Geometry check sheet. Reference: the model listing, model coordinates, mm. Face numbers are marked on the shaded views. A direction names the side the tool comes from. Coordinates: 2 decimals unless noted, no trailing zeros. Loops run counter-clockwise (first coordinate to the right, second up) from the corner with the lowest first, then second, coordinate; pieces in that order, holes last. Notation, with made-up numbers: M 66.25,77.25 L 112.25,77.25 A14 ccw 112.25,88.25 Z; hole C 64.25,87 d10. An arc over 180 degrees is marked long. Use CSV: the item, a comma, the result in double quotes.
Autodesk Fusion 360 part; units mm, degrees
sketch "mainBase" plane through (0, 0, 0) normal (0, 0, 1) x (1, 0, 0)
  line L0 (0, 0) -> (13.7, 0)
  line L1 (13.7, 0) -> (13.7, 6)
  line L2 (13.7, 6) -> (0, 6)
  line L3 (0, 6) -> (0, 0)
  line L4 (0, 0) -> (6.85, 0)
  line L5 (6.85, 0) -> (6.85, 1.75)
  line L6 (6.85, 1.75) -> (1.85, 1.75)
  line L7 (6.85, 1.75) -> (11.85, 1.75)
  line L8 (0, 6) -> (6.85, 6)
  circle A0 centre (1.85, 1.75) radius 1
  circle A1 centre (11.85, 1.75) radius 1
  line L9 (6.85, 6) -> (3.35, 6)
  line L10 (3.35, 6) -> (3.35, 2)
  line L11 (3.35, 2) -> (6.85, 2)
  line L12 (6.85, 2) -> (6.85, 6)
  line L13 (6.85, 6) -> (10.35, 6)
  line L14 (10.35, 6) -> (10.35, 2)
  line L15 (10.35, 2) -> (6.85, 2)
  line L16 (6.85, 2) -> (6.85, 6)
  dimension "d9" = 6
  dimension "d10" = 13.7
  dimension "d11" = 6.85
  dimension "d12" = 1.75
  dimension "d13" = 5
  dimension "d14" = 5
  dimension "d15" = 6.85
  dimension "d17" = 2
  dimension "d18" = 2
  dimension "d19" = 4
  dimension "d20" = 3.5
  dimension "d21" = 4
  dimension "d22" = 3.5
extrude "Extrude1" add sketch "mainBase" along normal blind 7.6 contours L2 L8 L9 L10 L11 L12 L16 | L2 L12 L13 L14 L15 L16
shell "Shell1" thickness 1 removed faces 1 at (5.6833, 4.6667, 0)
extrude "Extrude2" add sketch "mainBase" along normal blind 2 contours L0 L1 L2 L3 L4 L8 L10 L11 L14 L15
sketch "hallCutOut" plane through (0, 0, 0) normal (0, 0, 1) x (1, 0, 0)
  line L0 (0, 6) -> (6.85, 6)
  line L1 (6.85, 6) -> (6.85, 2)
  line L2 (6.85, 2) -> (3.35, 2)
  line L3 (3.35, 2) -> (3.35, 4)
  line L4 (6.85, 2) -> (6.85, 3)
  line L5 (6.85, 3) -> (5.95, 3)
  line L6 (5.95, 3) -> (3.35, 4)
  line L7 (6.85, 3) -> (7.75, 3)
  line L8 (6.85, 2) -> (10.35, 2)
  line L9 (10.35, 2) -> (10.35, 4)
  line L10 (10.35, 4) -> (7.75, 3)
  line L11 (7.75, 3) -> (9.35, 3)
  line L12 (9.35, 3) -> (9.35, 3.6154)
  line L13 (5.95, 3) -> (4.35, 3)
  line L14 (4.35, 3) -> (4.35, 3.6154)
  line L15 (6.85, 5) -> (8.95, 5)
  line L16 (8.95, 5) -> (8.95, 3)
  line L17 (8.95, 3) -> (6.85, 3)
  line L18 (6.85, 3) -> (6.85, 5)
  line L19 (6.85, 5) -> (4.75, 5)
  line L20 (4.75, 5) -> (4.75, 3)
  line L21 (4.75, 3) -> (6.85, 3)
  line L22 (6.85, 3) -> (6.85, 5)
  line L23 (9.35, 3) -> (4.35, 3)
  line L24 (4.35, 3) -> (4.35, 5)
  line L25 (4.35, 5) -> (9.35, 5)
  line L26 (9.35, 5) -> (9.35, 3)
  dimension "d31" = 6.85
  dimension "d32" = 4
  dimension "d33" = 3.5
  dimension "d34" = 2
  dimension "d35" = 1
  dimension "d36" = 0.9
  dimension "d37" = 0.9
  dimension "d38" = 3.5
  dimension "d39" = 2
  dimension "d59" = 2.1
extrude "Extrude3" add sketch "hallCutOut" along normal blind 6.6 contours L6 L13 L20 L21 L23 | L10 L11 L16 L17 L23 | L10 L11 L12 L16 L23 L26 | L6 L13 L14 L20 L23 L24
sketch "wireCutOut" plane through (0, 0, 0) normal (0, -1, 0) x (1, 0, 0)
  line L0 (0, 0) -> (13.7, 0)
  line L1 (13.7, 0) -> (13.7, 2)
  line L2 (13.7, 2) -> (0, 2)
  line L3 (0, 2) -> (0, 0)
  line L4 (0, 0) -> (6.85, 0)
  line L5 (6.85, 0) -> (6.85, 1)
  line L6 (6.85, 1) -> (5.95, 1)
  line L7 (6.85, 1) -> (7.75, 1)
  line L8 (6.85, 0) -> (13.7, 0)
  line L9 (6.85, 0) -> (10.35, 0)
  line L10 (6.85, 0) -> (3.35, 0)
  line L11 (7.75, 1) -> (10.35, 0)
  line L12 (5.95, 1) -> (3.35, 0)
  dimension "d42" = 6.85
  dimension "d43" = 1
  dimension "d44" = 0.9
  dimension "d45" = 0.9
  dimension "d46" = 6.85
  dimension "d47" = 3.5
  dimension "d48" = 3.5
extrude "Extrude4" cut sketch "wireCutOut" against normal blind 5 contours L0 L4 L5 L6 L10 L12 | L0 L5 L7 L8 L9 L11
sketch "cutOut" plane through (0, 0, 0) normal (0, 0, 1) x (1, 0, 0)
  line L0 (0, 0) -> (13.7, 0)
  line L1 (13.7, 0) -> (13.7, 6)
  line L2 (13.7, 6) -> (0, 6)
  line L3 (0, 6) -> (0, 0)
  line L4 (13.7, 0) -> (13.7, 2)
  line L5 (0, 0) -> (0, 2)
  line L6 (0, 6) -> (2, 6)
  line L7 (13.7, 6) -> (11.7, 6)
  line L8 (0, 2) -> (2, 6)
  line L9 (13.7, 2) -> (11.7, 6)
  dimension "d51" = 6
  dimension "d52" = 13.7
  dimension "d53" = 2
  dimension "d54" = 2
  dimension "d55" = 2
  dimension "d56" = 2
extrude "Extrude5" cut sketch "cutOut" along normal blind 2 contours L2 L3 L6 L8 | L1 L2 L7 L9
extrude "Extrude6" add sketch "hallCutOut" along normal blind 7.6 contours L10 L16 L25 L26 | L6 L20 L24 L25
extrude "Extrude7" cut sketch "wireCutOut" against normal blind 5 contours L0 L4 L5 L6 L10 L12 | L0 L5 L7 L8 L9 L11
extrude "Extrude8" cut sketch "hallCutOut" along normal blind 6.6 contours L10 L16 L25 L26 | L6 L20 L24 L25
equation "baseLength = 6 mm"
equation "baseWidth = 13.7 mm"
equation "mountingCircleToMountingCircle = 10 mm"
equation "mountingHoleFromEdge = 1.75 mm"
equation "hallEffectWidth = 7 mm"
equation "hallEffectLength = 4 mm"
equation "hallEffectHeight = 7.6 mm"
equation "baseHeight = 2 mm"
equation "d9 = baseLength"
equation "d10 = baseWidth"
equation "d11 = baseWidth / 2"
equation "d12 = mountingHoleFromEdge"
equation "d13 = mountingCircleToMountingCircle / 2"
equation "d14 = mountingCircleToMountingCircle / 2"
equation "d15 = baseWidth / 2"
equation "screwHole = 2 mm"
equation "d17 = screwHole"
equation "d18 = screwHole"
equation "d19 = hallEffectLength"
equation "d20 = hallEffectWidth / 2"
equation "d21 = hallEffectLength"
equation "d22 = hallEffectWidth / 2"
equation "d23 = hallEffectHeight"
equation "hallEffectThickness = 1 mm"
equation "d26 = hallEffectThickness"
equation "d27 = baseHeight"
equation "traingleHeight = 2 mm"
equation "hallEffectMiddleDist = 1.8 mm"
equation "d31 = baseWidth / 2"
equation "d32 = hallEffectLength"
equation "d33 = hallEffectWidth / 2"
equation "d34 = traingleHeight"
equation "d35 = hallEffectThickness"
equation "d36 = hallEffectMiddleDist / 2"
equation "d37 = hallEffectMiddleDist / 2"
equation "d38 = hallEffectWidth / 2"
equation "d39 = traingleHeight"
equation "d40 = hallEffectHeight - hallEffectThickness"
equation "d42 = baseWidth / 2"
equation "d43 = hallEffectThickness"
equation "d44 = hallEffectMiddleDist / 2"
equation "d45 = hallEffectMiddleDist / 2"
equation "d46 = baseWidth / 2"
equation "d47 = hallEffectWidth / 2"
equation "d48 = hallEffectWidth / 2"
equation "d51 = baseLength"
equation "d52 = baseWidth"
equation "d53 = baseLength / 3"
equation "d54 = baseLength / 3"
equation "d57 = baseHeight"
equation "d60 = hallEffectHeight"
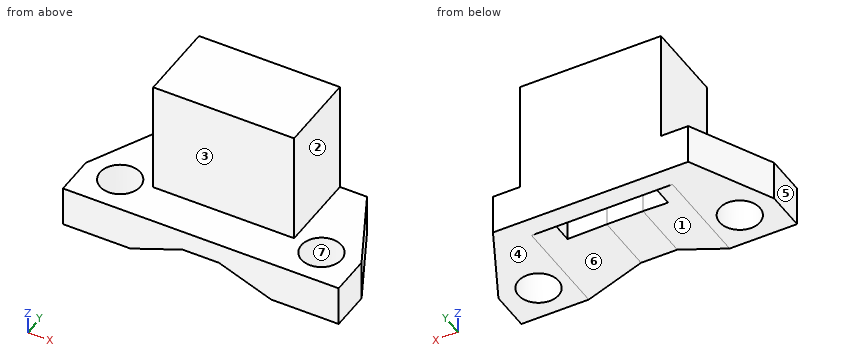
1. Release check for a two-part mould opening along X. For the marked faces 4, 5, 6 and 7 record: +X half, -X half, draft (parallel to the pull), parting line (faces both ways), or undercut.
The answers:
face 4,"draft"
face 5,"-X half"
face 6,"undercut"
face 7,"undercut"
2. Section check D-D, the plane z = 5.75. Record the cut outline in (x, y), plus the area to 3 significant figures.
The answers:
outline,"M 3.35,2 L 10.35,2 L 10.35,6 L 3.35,6 Z; hole M 4.35,3.62 L 5.95,3 L 7.75,3 L 9.35,3.62 L 9.35,5 L 4.35,5 Z"
area,"19.0 mm^2"
3. Gauge pin test, flat ends, axial feed: P1, Ø1.7, axis at x = 6, z = 6, coming from the -Y side; P2, Ø1.4, axis at x = 7, y = 1.5, coming from the -Z side; P3, Ø1.6, axis at x = 1.85, y = 1.75, coming from the +Z side; P4, Ø1, axis at x = 6, y = 4, coming from the -Z side. Record the tip position at first contact, or that the pin passes through.
The answers:
P1,"y = 2"
P2,"z = 1"
P3,"through"
P4,"z = 6.6"
4. Section check C-C, the plane x = 6.25. Record the cut outline in (y, z).
The answers:
outline,"M 0,1 L 3,1 L 3,6.6 L 5,6.6 L 5,0 L 6,0 L 6,7.6 L 2,7.6 L 2,2 L 0,2 Z"
5. Section check B-B, the plane x = 11.25. Record the cut outline in (y, z), plus the area to 3 significant figures.
The answers:
outline,"M 0,0 L 0.95,0 L 0.95,2 L 0,2 Z; M 2.55,0 L 6,0 L 6,2 L 2.55,2 Z"
area,"8.80 mm^2"
6. Section check A-A, the plane y = 1.75. Record the cut outline in (x, z), plus the area to 3 significant figures.
The answers:
outline,"M 0,0 L 0.85,0 L 0.85,2 L 0,2 Z; M 2.85,0 L 3.35,0 L 5.95,1 L 7.75,1 L 10.35,0 L 10.85,0 L 10.85,2 L 2.85,2 Z; M 12.85,0 L 13.7,0 L 13.7,2 L 12.85,2 Z"
area,"15.0 mm^2"
7. Set-up check for the marked faces 1, 2 and 3: record each of +Z, -Z, +X, -X, +Y, -Y from which the full face is reachable in a straight line by a thin tool's end or side.
The answers:
face 1,"-Z, -Y"
face 2,"+Z, +X, +Y, -Y"
face 3,"+Z, +X, -X, -Y"
8. Thickness scan on line 1 (X direction, y = 1.8, z = 1.5); line 2 (X direction, y = 4.55, z = 4.5); line 3 (Y direction, x = 7, z = 1.5). Record the ranges inside material, lowest first. Write a range as [from, to].
The answers:
line 1,"[0, 0.85], [2.85, 10.85], [12.85, 13.7]"
line 2,"[3.35, 4.35], [9.35, 10.35]"
line 3,"[0, 3], [5, 6]"
